For this review, take the finished solid that the model builds, in its own axes (mm). Face numbers are marked on the shaded views. A direction names the side the tool comes from. Round coordinates to 2 decimals unless told otherwise and drop trailing zeros. Order: outer loops, then holes, each group sorted by start corner. A loop starts at its lowest first (then second) coordinate and runs counter-clockwise, first axis right, second up. Notation, with made-up numbers: (84.5, 34) - (143.5, 34) arc R28 cw to (143.5, 52) - close; hole circle Ø1 at (49.5, -33.75). An arc over 180 degrees is marked (long way). Write each question's results on one line, items separated by ' | '. Start each with the question number.
(1) Insertion check: pin 1 Ø7 at (x, z) = (0, -17) entering from +Y; pin 2 Ø5 at (x, z) = (0, 17) entering from +Y; pin 3 Ø3 at (x, y) = (-3, 2) entering from -Z; pin 4 Ø4 at (x, z) = (-0.5, 0.5) entering from -Y. Each pin has a flat end and moves straight along its axis. Give the tip position at first contact, or say it passes through.
(2) Take a section at C-C, the plane z = -13.5. Give the boundary of the cut face in (x, y).
(3) Draft analysis for pull direction Z (two halves, no side actions). For the marked faces 1, 2 and 3, state which applies: pulls with the +Z half, pulls with the -Z half, needs draft (parallel to the pull), parting line crosses it, or undercut.
(4) Take a section at B-B, the plane y = -0.75. Give the boundary of the cut face in (x, z), plus the area to 3 significant figures.
(5) Take a section at A-A, the plane x = 1.25. Give the boundary of the cut face in (y, z), plus the area to 3 significant figures.
(6) Take a section at D-D, the plane x = -2. Give the boundary of the cut face in (y, z).
(7) For the marked faces 4, 5 and 6, list the 3-axis set-ups (+Z, -Z, +X, -X, +Y, -Y) from which the entire face can be reached by the end or side of a thin tool; tool diameter is ignored.
(8) For L1, parallel to Z at x = 0, y = -3.6; L2, parallel to X at y = -4.2, z = 17; L3, parallel to Z at x = 0, y = -3.1, list the stretches that pass through material, from the lowest coordinate up. Write a range as from..to.
Autodesk Inventor part; units mm, degrees
ref_plane "YZ Plane" through (0, 0, 0) normal (1, 0, 0) x (0, 1, 0)
ref_plane "XZ Plane" through (0, 0, 0) normal (0, 1, 0) x (-1, 0, 0)
ref_plane "XY Plane" through (0, 0, 0) normal (0, 0, 1) x (1, 0, 0)
sketch "Sketch1" plane through (0, 0, 0) normal (0, 1, 0) x (-1, 0, 0)
  line L0 (-6, 4) -> (6, 4)
  line L1 (6, 4) -> (6, -4)
  line L2 (6, -4) -> (-6, -4)
  line L3 (-6, -4) -> (-6, 4)
  line L4 (-6, 4) -> (6, -4) construction
  line L5 (6, 4) -> (-6, -4) construction
  point P0 (0, 0)
  dimension "d0" = 12
  dimension "d1" = 8
extrude "Plate1" add sketch "Sketch1" along normal blind 3.2
sketch "Sketch2" plane through (-6, -0.3547, -4.9745) normal (0, 0.7660444, -0.6427876) x (1, 0, 0)
  line L0 (12, 0) -> (0, 0)
  line L1 (0, 0) -> (0, -5.8835)
  line L2 (0, -5.8835) -> (12, -5.8835)
  line L3 (12, -5.8835) -> (12, 0)
edge flange "Flange1" height 7.6 angle 40 thickness 3.2 bend radius 1.516 thickness toward (0, 0.7660444, -0.6427876) relief tear relief width 3.2 relief depth 1.6 edges at (0, 3.2, -4) wall of the first edge with corners at (6, -0.3547, -4.9745) (-6, -0.3547, -4.9745) (-6, -4.1365, -9.4815) (6, -4.1365, -9.4815)
bend "Bend1"
corner "Corner1"
sketch "Sketch3" plane through (6, -2.0399, -12.5129) normal (0, -1, 0) x (-1, 0, 0)
  line L0 (12, 0) -> (0, 0)
  line L1 (0, 0) -> (0, -10.2835)
  line L2 (0, -10.2835) -> (12, -10.2835)
  line L3 (12, -10.2835) -> (12, 0)
edge flange "Flange2" height 12 angle 40 thickness 3.2 bend radius 1.516 thickness toward (0, -1, 0) relief tear relief width 3.2 relief depth 1.6 edges at (0, -4.1365, -9.4815) wall of the first edge with corners at (-6, -2.0399, -12.5129) (6, -2.0399, -12.5129) (6, -2.0399, -22.7964) (-6, -2.0399, -22.7964)
bend "Bend2"
corner "Corner2"
sketch "Sketch4" plane through (6, -0.3547, 4.9745) normal (0, 0.7660444, 0.6427876) x (1, 0, 0)
  line L0 (-12, 0) -> (0, 0)
  line L1 (0, 0) -> (0, 5.8835)
  line L2 (0, 5.8835) -> (-12, 5.8835)
  line L3 (-12, 5.8835) -> (-12, 0)
edge flange "Flange3" height 7.6 angle 40 thickness 3.2 bend radius 1.516 thickness toward (0, 0.7660444, 0.6427876) relief tear relief width 3.2 relief depth 1.6 edges at (0, 3.2, 4) wall of the first edge with corners at (-6, -0.3547, 4.9745) (6, -0.3547, 4.9745) (6, -4.1365, 9.4815) (-6, -4.1365, 9.4815)
bend "Bend3"
corner "Corner3"
sketch "Sketch5" plane through (-6, -2.0399, 12.5129) normal (0, -1, 0) x (-1, 0, 0)
  line L0 (-12, 0) -> (0, 0)
  line L1 (0, 0) -> (0, 10.2835)
  line L2 (0, 10.2835) -> (-12, 10.2835)
  line L3 (-12, 10.2835) -> (-12, 0)
edge flange "Flange4" height 12 angle 40 thickness 3.2 bend radius 1.516 thickness toward (0, -1, 0) relief tear relief width 3.2 relief depth 1.6 edges at (0, -4.1365, 9.4815) wall of the first edge with corners at (6, -2.0399, 12.5129) (-6, -2.0399, 12.5129) (-6, -2.0399, 22.7964) (6, -2.0399, 22.7964)
bend "Bend4"
corner "Corner4"
fillet "Fillet1" radius 6 4 edges at (6, -3.6399, -22.7964) (-6, -3.6399, -22.7964) (6, -3.6399, 22.7964) (-6, -3.6399, 22.7964)
sketch "Sketch6" plane through (-6, -2.0399, 12.5129) normal (0, 1, 0) x (1, 0, 0)
  arc A0 (0, -4.2835) -> (12, -4.2835) centre (6, -4.2835) ccw
  line L0 (6, -10.2835) -> (6, 35.3093)
  arc A1 (12, 29.3093) -> (0, 29.3093) centre (6, 29.3093) ccw
  line L1 (6, 12.5129) -> (6, -4.4871)
  circle A2 centre (6, -4.4871) radius 3
  line L2 (6, 12.5129) -> (6, 29.5129)
  circle A3 centre (6, 29.5129) radius 3
  dimension "d50" = 17
  dimension "d51" = 6
  dimension "d52" = 17
  dimension "d53" = 6
extrude "Cut1" cut sketch "Sketch6" against normal blind 3.2
equation "\"d54\" = Thickness"
equation "\"d2\" = Thickness"
equation "\"d3\" = BendReliefWidth"
equation "\"d4\" = BendReliefDepth"
equation "\"d5\" = MinimumRemnant"
equation "\"d6\" = TransitionRadius"
equation "\"d9\" = BendRadius"
equation "\"d10\" = CornerReliefSize"
equation "\"d11\" = GapSize"
equation "\"d12\" = JacobiRadiusSize"
equation "\"d13\" = BendReliefWidth"
equation "\"d14\" = BendReliefDepth"
equation "\"d15\" = MinimumRemnant"
equation "\"d16\" = TransitionRadius"
equation "\"d19\" = BendRadius"
equation "\"d20\" = CornerReliefSize"
equation "\"d21\" = GapSize"
equation "\"d22\" = JacobiRadiusSize"
equation "\"d23\" = BendReliefWidth"
equation "\"d24\" = BendReliefDepth"
equation "\"d25\" = MinimumRemnant"
equation "\"d26\" = TransitionRadius"
equation "\"d29\" = BendRadius"
equation "\"d30\" = CornerReliefSize"
equation "\"d31\" = GapSize"
equation "\"d32\" = JacobiRadiusSize"
equation "\"d33\" = BendReliefWidth"
equation "\"d34\" = BendReliefDepth"
equation "\"d35\" = MinimumRemnant"
equation "\"d36\" = TransitionRadius"
equation "\"d39\" = BendRadius"
equation "\"d40\" = CornerReliefSize"
equation "\"d41\" = GapSize"
equation "\"d42\" = JacobiRadiusSize"
equation "\"BendReliefWidth\" = Thickness"
equation "\"BendReliefDepth\" = 0.5 * Thickness"
equation "\"CornerReliefSize\" = 4 * Thickness"
equation "\"MinimumRemnant\" = 2 * Thickness"
equation "\"TransitionRadius\" = BendRadius"
equation "\"JacobiRadiusSize\" = BendRadius"
equation "\"GapSize\" = Thickness"
properties part number "SP7V1 Viela Freno" material "Stainless Steel"
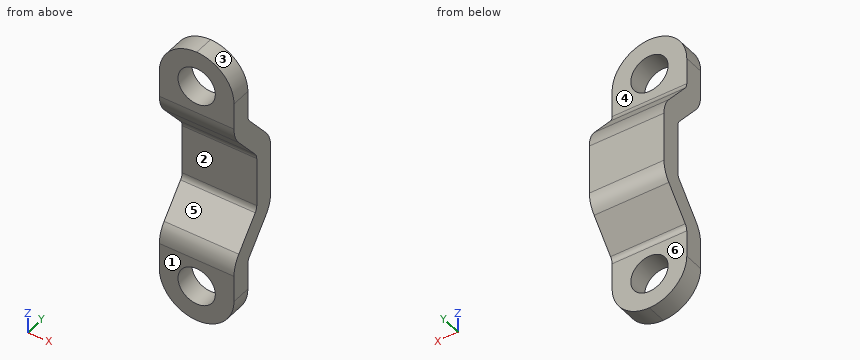
Results below:
1) pin 1: stops at y = -2.04 | pin 2: passes through | pin 3: stops at z = -8.93 | pin 4: stops at y = 0
2) outline: (-6, -5.24) - (6, -5.24) - (6, -2.04) - (-6, -2.04) - close
3) face 1: needs draft | face 2: undercut | face 3: pulls with the +Z half
4) outline: (-6, -10.42) - (6, -10.42) - (6, -5.45) - (-6, -5.45) - close; (-6, 5.45) - (6, 5.45) - (6, 10.42) - (-6, 10.42) - close | area: 119 mm^2
5) outline: (-5.24, -22.66) - (-2.04, -22.66) - (-2.04, -19.73) - (-5.24, -19.73) - close; (-5.24, -14.27) - (-2.04, -14.27) - (-2.04, -12.51) arc R1.52 cw to (-1.69, -11.54) - (2.1, -7.03) arc R4.72 ccw to (3.2, -4) - (3.2, 4) arc R4.72 ccw to (2.1, 7.03) - (-1.69, 11.54) arc R1.52 cw to (-2.04, 12.51) - (-2.04, 14.27) - (-5.24, 14.27) - (-5.24, 12.51) arc R4.72 ccw to (-4.14, 9.48) - (-0.35, 4.97) arc R1.52 cw to (0, 4) - (0, -4) arc R1.52 cw to (-0.35, -4.97) - (-4.14, -9.48) arc R4.72 ccw to (-5.24, -12.51) - close; (-5.24, 19.73) - (-2.04, 19.73) - (-2.04, 22.66) - (-5.24, 22.66) - close | area: 121 mm^2
6) outline: (-5.24, -22.45) - (-2.04, -22.45) - (-2.04, -19.24) - (-5.24, -19.24) - close; (-5.24, -14.76) - (-2.04, -14.76) - (-2.04, -12.51) arc R1.52 cw to (-1.69, -11.54) - (2.1, -7.03) arc R4.72 ccw to (3.2, -4) - (3.2, 4) arc R4.72 ccw to (2.1, 7.03) - (-1.69, 11.54) arc R1.52 cw to (-2.04, 12.51) - (-2.04, 14.76) - (-5.24, 14.76) - (-5.24, 12.51) arc R4.72 ccw to (-4.14, 9.48) - (-0.35, 4.97) arc R1.52 cw to (0, 4) - (0, -4) arc R1.52 cw to (-0.35, -4.97) - (-4.14, -9.48) arc R4.72 ccw to (-5.24, -12.51) - close; (-5.24, 19.24) - (-2.04, 19.24) - (-2.04, 22.45) - (-5.24, 22.45) - close
7) face 4: +Z, +X, -X, +Y | face 5: +X, -X, -Y | face 6: -Z, +X, -X, +Y
8) L1: z = -22.8..-20, -14..-8.84, 8.84..14, 20..22.8 | L2: x = -6..-3, 3..6 | L3: z = -22.8..-20, -14..-8.25, 8.25..14, 20..22.8
